from build123d import *

# Parameters (mm, degrees)
BOSS_EXTRUDE1_DEPTH = 17.5
BOSS_EXTRUDE2_DEPTH = 5
CUT_EXTRUDE1_DEPTH  = 97.898655256
CUT_EXTRUDE2_DEPTH  = 97.898655256
CUT_EXTRUDE3_DEPTH  = 97.898655256
CUT_EXTRUDE4_DEPTH  = 97.898655256
SKETCH7_W           = 20.085317587
SKETCH7_H           = 17.517779008
CUT_EXTRUDE5_DEPTH  = 97.898655256
HOLE1_D             = 3.4
HOLE2_D             = 8.4
HOLE3_D             = 4.4
HOLE4_D             = 23
HOLE5_D             = 8.4
HOLE6_D             = 4.4
FILLET1_R           = 8
CHAMFER3_SIZE       = 4
CHAMFER4_SIZE       = 2
FILLET2_R           = 5
FILLET3_R           = 9
FILLET4_R           = 9


with BuildPart() as part:
    # Sketch1 → Boss-Extrude1 (new body)
    with BuildSketch(Plane(origin=(0, 0, 0), x_dir=(0, -1, 0), z_dir=(-1, 0, 0))):
        with BuildLine():
            Line((11.200465877, 72.380538081), (-8.757531911, 37.812271895))
            ThreePointArc((-8.757531911, 37.812271895), (-19.547871207, 38.906001768), (-24.988655697, 29.523809524))
            Line((-24.988655697, 29.523809524), (-23.581163303, 0))
            Line((-23.581163303, 0), (46.605341047, 0))
            Line((46.605341047, 0), (62.001266902, 42.299958639))
            Line((62.001266902, 42.299958639), (11.200465877, 72.380538081))
        make_face()
    extrude(amount=-BOSS_EXTRUDE1_DEPTH)

    # Sketch2 → Boss-Extrude2 (add)
    with BuildSketch(Plane(origin=(0, 0, 0), x_dir=(0, -1, 0), z_dir=(-1, 0, 0))):
        with BuildLine():
            Line((-8.757531911, 37.812271895), (3.302003533, 58.7))
            Line((3.302003533, 58.7), (-12, 58.7))
            Line((-12, 58.7), (-12, 39.539392014))
            ThreePointArc((-12, 39.539392014), (-10.298772493, 38.82601042), (-8.757531911, 37.812271895))
        make_face()
    extrude(amount=-BOSS_EXTRUDE2_DEPTH)

    # Sketch3 → Cut-Extrude1 (cut, through all)
    with BuildSketch(Plane.ZY):
        with BuildLine():
            Line((18.944189974, -15.937202057), (20.438371168, -19.141483967))
            ThreePointArc((20.438371168, -19.141483967), (22.697545451, -19.96375616), (23.519817644, -17.704581878))
            Line((23.519817644, -17.704581878), (22.02563645, -14.500299967))
            ThreePointArc((22.02563645, -14.500299967), (19.766462167, -13.678027774), (18.944189974, -15.937202057))
        make_face()
    extrude(amount=-CUT_EXTRUDE1_DEPTH, mode=Mode.SUBTRACT)

    # Sketch4 → Cut-Extrude2 (cut, through all)
    with BuildSketch(Plane.ZY):
        with BuildLine():
            Line((48.896933411, -24.280652217), (45.692651501, -25.774833411))
            ThreePointArc((45.692651501, -25.774833411), (44.870379308, -28.034007694), (47.129553591, -28.856279887))
            Line((47.129553591, -28.856279887), (50.333835501, -27.362098693))
            ThreePointArc((50.333835501, -27.362098693), (51.156107694, -25.10292441), (48.896933411, -24.280652217))
        make_face()
    extrude(amount=-CUT_EXTRUDE2_DEPTH, mode=Mode.SUBTRACT)

    # Sketch5 → Cut-Extrude3 (cut, through all)
    with BuildSketch(Plane.ZY):
        with BuildLine():
            Line((35.977855582, -52.466015834), (37.472036775, -55.670297745))
            ThreePointArc((37.472036775, -55.670297745), (39.731211058, -56.492569938), (40.553483251, -54.233395655))
            Line((40.553483251, -54.233395655), (39.059302058, -51.029113744))
            ThreePointArc((39.059302058, -51.029113744), (36.800127775, -50.206841551), (35.977855582, -52.466015834))
        make_face()
    extrude(amount=-CUT_EXTRUDE3_DEPTH, mode=Mode.SUBTRACT)

    # Sketch6 → Cut-Extrude4 (cut, through all)
    with BuildSketch(Plane.ZY):
        with BuildLine():
            Line((10.600739814, -45.889945495), (13.805021724, -44.395764301))
            ThreePointArc((13.805021724, -44.395764301), (14.627293917, -42.136590018), (12.368119634, -41.314317825))
            Line((12.368119634, -41.314317825), (9.163837724, -42.808499019))
            ThreePointArc((9.163837724, -42.808499019), (8.341565531, -45.067673302), (10.600739814, -45.889945495))
        make_face()
    extrude(amount=-CUT_EXTRUDE4_DEPTH, mode=Mode.SUBTRACT)

    # Sketch7 → Cut-Extrude5 (cut, through all)
    with BuildSketch(Plane(origin=(17.5, 0, 0), x_dir=(0, 0, -1), z_dir=(1, 0, 0))):
        with Locations((-19.957341207, -0.762832283)):
            Rectangle(SKETCH7_W, SKETCH7_H)
    extrude(amount=-CUT_EXTRUDE5_DEPTH, mode=Mode.SUBTRACT)

    # Hole1 (through all)
    with Locations(Plane(origin=(5, 0, 0), x_dir=(0, 0, -1), z_dir=(1, 0, 0))):
        with Locations((-50.7, 7)):
            Hole(HOLE1_D / 2)

    # Hole2 (through all)
    with Locations(Plane.ZY):
        with Locations((9, 15)):
            Hole(HOLE2_D / 2)

    # Hole3 (through all)
    with Locations(Plane.ZY):
        with Locations((40.5, -12.150669091)):
            Hole(HOLE3_D / 2)

    # Hole4 (through all)
    with Locations(Plane.ZY):
        with Locations((29.748836613, -35.085298856)):
            Hole(HOLE4_D / 2)

    # Hole5 (through all)
    with Locations(Plane.ZY):
        with Locations((60, -14.444863729)):
            Hole(HOLE5_D / 2)

    # Hole6 (through all)
    with Locations(Plane.ZY):
        with Locations((30, 15)):
            Hole(HOLE6_D / 2)

    # Fillet1
    fillet1_edges = [part.edges().sort_by_distance(p)[0] for p in [
        (11.25, 8.757531911, 37.812271895),
    ]]
    fillet(fillet1_edges, radius=FILLET1_R)

    # Chamfer3
    chamfer3_edges = [part.edges().sort_by_distance(p)[0] for p in [
        (2.5, 12, 58.7),
    ]]
    chamfer(chamfer3_edges, length=CHAMFER3_SIZE)

    # Chamfer4
    chamfer4_edges = [part.edges().sort_by_distance(p)[0] for p in [
        (8.75, 7.996057221, 9.914682413),
    ]]
    chamfer(chamfer4_edges, length=CHAMFER4_SIZE)

    # Fillet2
    fillet2_edges = [part.edges().sort_by_distance(p)[0] for p in [
        (8.75, -62.001266902, 42.299958639),
    ]]
    fillet(fillet2_edges, radius=FILLET2_R)

    # Fillet3
    fillet3_edges = [part.edges().sort_by_distance(p)[0] for p in [
        (8.75, -11.200465877, 72.380538081),
    ]]
    fillet(fillet3_edges, radius=FILLET3_R)

    # Fillet4
    fillet4_edges = [part.edges().sort_by_distance(p)[0] for p in [
        (8.75, 23.581163303, 0),
    ]]
    fillet(fillet4_edges, radius=FILLET4_R)


solid = part.part
Could you check a few things on this model? Use its own coordinates, in mm. A direction names the side the tool comes from. Coordinates: 2 decimals unless noted, no trailing zeros. Write each loop counter-clockwise with the first axis right and the second up, starting at its lowest first coordinate (ties: lowest second). Pieces come first, ordered by that corner, then holes. Notation, with made-up numbers: (62, 4) - (107, 4) arc R32 ccw to (107, 30) - close; hole circle Ø9 at (-26.5, 11). An arc over 180 degrees is marked (long way). Put each result on its own line as item: value. Start each with the question number.
Q1. Please list where these lines run through material, in increasing order: L1, parallel to Y at x = 14.5, z = 39; L2, parallel to Z at x = 7, y = -45.5; L3, parallel to Z at x = 9.25, y = -43.
Q2. I want a section at D-D on x = 3.75. Count the separate pieces of the cut face and the enclosed holes in it, plus the area to 3 significant figures.
Q3. I want a section at C-C on y = 7. Write out the boundary of the cut face in (x, z), plus the area to 3 significant figures.
Q4. Which directions (+Z, -Z, +X, -X, +Y, -Y) give clear straight access to the entire face, cutting with the end or side of a thin tool? Please do faces 4 (the flat face through (8.628, -25.017, 47.317)), 5 (the flat face through (2, 2, 58.7)), 6 (the flat face through (8.628, -53.496, 18.932)).
Q5. Thinking about a two-plate mould opening in Z: for faces 1 (the flat face through (0, -17, 27)), 2 (the cylindrical face through (8.872, 15.097, 32.198)), 3 (the flat face through (8.628, 24.496, 19.194)), which applies, pulls with the +Z half, pulls with the -Z half, needs draft (parallel to the pull), parting line crosses it, or undercut?
Q6. I'm going to push flat-ended pins straight in: P1, Ø7.5, axis at y = -14.44, z = 60, coming from the +X side; P2, Ø10, axis at x = 14, z = 31.5, coming from the -Y side; P3, Ø1.5, axis at x = 13, z = 57, coming from the +Y side; P4, Ø1.5, axis at x = 3.5, z = 51, coming from the +Y side. Where does each tip first touch, or does it pass through?
Q7. I want a section at B-B on y = -2. Write out the boundary of the cut face in (x, z), plus the area to 3 significant figures.
Q8. I want a section at A-A on z = 57.5. Write out the boundary of the cut face in (x, y), plus the area to 3 significant figures.
Checks:
1. L1: -60.76 to -56.65, -50.91 to -41.92, -28.25 to -13.76, -10.54 to 19.36
1. L2: 0 to 8.63, 11.44 to 24.87, 34.63 to 52.07
1. L3: 0 to 8.85, 14.78 to 21.41, 38.09 to 53.55
2. separate pieces: 1
2. enclosed holes: 11
2. area: 3,440 mm²
3. outline: (0, 0) - (17.5, 0) - (17.5, 10.92) - (0, 10.92) - close; (0, 30) - (17.5, 30) - (17.5, 41.74) - (5, 41.74) - (5, 49) - (0, 49) - close; (0, 52.4) - (5, 52.4) - (5, 58.7) - (0, 58.7) - close
3. area: 464 mm²
4. face 4: +X, -X
4. face 5: +Z, +X, -X, +Y
4. face 6: -Z, +X, -X, -Y
5. face 1: needs draft
5. face 2: undercut
5. face 3: pulls with the -Z half
6. P1: through
6. P2: y = -59.89
6. P3: y = -1.89
6. P4: y = 12
7. outline: (0, 0) - (17.5, 0) - (17.5, 9.91) - (0, 9.91) - close; (0, 30) - (17.5, 30) - (17.5, 56.44) - (5, 56.44) - (5, 58.7) - (0, 58.7) - close
7. area: 648 mm²
8. outline: (0, -36.33) - (17.5, -36.33) - (17.5, -17.82) - (0, -17.82) - close; (0, -11.07) - (17.5, -11.07) - (17.5, -2.61) - (5, -2.61) - (5, 9.2) - (0, 9.2) - close
8. area: 531 mm²
